Work out the finished part from the listing and answer in its coordinate system (mm). Face numbers are marked on the shaded views. Give positions to 0.01 mm unless a question says otherwise; leave off trailing zeros. Order: outer loops, then holes, each group sorted by start corner. A loop starts at its lowest first (then second) coordinate and runs counter-clockwise, first axis right, second up. Notation, with made-up numbers: (-1.75, 7) - (11.25, 7) arc R29 cw to (11.25, 32) - close; hole circle Ø7 at (71, 71). An arc over 180 degrees is marked (long way). Put each result on its own line as item: value.
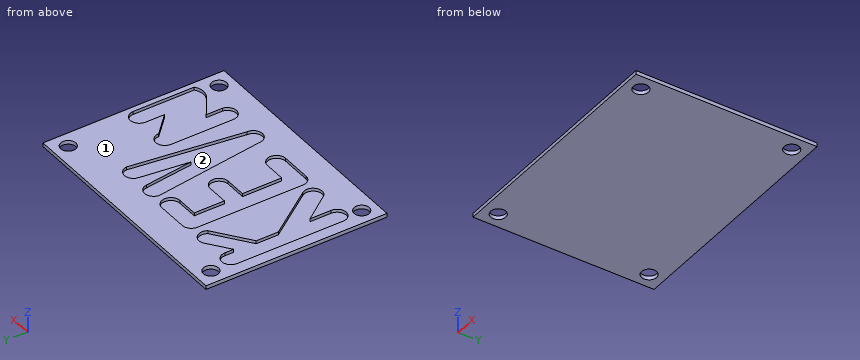
Autodesk Inventor part; units mm, degrees
ref_plane "YZ Plane" through (0, 0, 0) normal (1, 0, 0) x (0, 1, 0)
ref_plane "XZ Plane" through (0, 0, 0) normal (0, 1, 0) x (-1, 0, 0)
ref_plane "XY Plane" through (0, 0, 0) normal (0, 0, 1) x (1, 0, 0)
sketch "Sketch1" plane through (0, 0, 0) normal (0, 0, 1) x (1, 0, 0)
  line L0 (0, 0) -> (203.2, 0)
  line L1 (203.2, 0) -> (203.2, -152.4)
  line L2 (203.2, -152.4) -> (0, -152.4)
  line L3 (0, -152.4) -> (0, 0)
  line L4 (0, 0) -> (12.7, 0)
  line L5 (0, -12.7) -> (0, 0)
  line L6 (0, -152.4) -> (0, -139.7)
  line L7 (203.2, 0) -> (190.5, 0)
  line L8 (203.2, -152.4) -> (203.2, -139.7)
  circle A0 centre (12.7, -12.7) radius 6.35
  circle A1 centre (190.5, -12.7) radius 6.35
  circle A2 centre (190.5, -139.7) radius 6.35
  circle A3 centre (12.7, -139.7) radius 6.35
extrude "Extrusion1" add sketch "Sketch1" along normal blind 3.175
sketch "Sketch2" plane through (0, 0, 3.175) normal (0, 0, 1) x (1, 0, 0)
  arc A0 (24.817, -32.5655) -> (9.577, -32.5655) centre (17.197, -32.5655) ccw
  arc A1 (9.577, -122.0402) -> (24.817, -122.0402) centre (17.197, -122.0402) ccw
  line L0 (9.577, -32.5655) -> (9.577, -122.0402)
  line L1 (9.577, -42.2151) -> (9.577, -32.5655)
  arc A2 (53.0983, -37.3903) -> (42.7617, -26.7428) centre (46.6851, -33.275) ccw
  arc A3 (49.095, -40.7739) -> (42.7617, -26.7428) centre (46.7521, -33.3865) ccw
  line L2 (42.7617, -26.7428) -> (24.817, -40.0522)
  line L3 (53.0983, -37.3903) -> (24.3404, -58.7199)
  arc A4 (42.2851, -127.8629) -> (53.0983, -117.2154) centre (47.2004, -122.0402) ccw
  line L4 (53.0983, -117.2154) -> (24.3404, -77.3028)
  line L5 (42.2851, -127.8629) -> (24.817, -104.3113)
  line L6 (24.817, -104.3113) -> (24.817, -122.0402)
  line L7 (24.3404, -58.7199) -> (24.3404, -77.3028)
  line L8 (24.817, -40.0522) -> (24.817, -32.5655)
  line L9 (60.5227, -33.6636) -> (60.5227, -122.5636)
  line L10 (68.1427, -130.1836) -> (93.5427, -130.1836)
  line L11 (93.5427, -114.9436) -> (75.7627, -114.9436)
  line L12 (68.1427, -26.0436) -> (93.5427, -26.0436)
  line L13 (93.5427, -41.2836) -> (75.7627, -41.2836)
  arc A5 (68.1427, -26.0436) -> (60.5227, -33.6636) centre (68.1427, -33.6636) ccw
  arc A6 (60.5227, -122.5636) -> (68.1427, -130.1836) centre (68.1427, -122.5636) ccw
  arc A7 (93.5427, -130.1836) -> (93.5427, -114.9436) centre (93.5427, -122.5636) ccw
  arc A8 (93.5427, -41.2836) -> (93.5427, -26.0436) centre (93.5427, -33.6636) ccw
  arc A9 (93.5427, -81.8927) -> (93.5427, -66.6527) centre (93.5427, -74.2727) ccw
  line L14 (93.5427, -66.6527) -> (75.7627, -66.6527)
  line L15 (93.5427, -81.8927) -> (75.7627, -81.8927)
  line L16 (75.7627, -41.2836) -> (75.7627, -66.6527)
  line L17 (75.7627, -81.8927) -> (75.7627, -114.9436)
  line L18 (147.1171, -32.5701) -> (134.4171, -125.4887)
  line L19 (106.4768, -32.5655) -> (119.2541, -126.5682)
  line L20 (121.6953, -32.0671) -> (126.8219, -72.9902)
  line L21 (126.8219, -72.9902) -> (131.9604, -32.2167)
  arc A10 (147.1171, -32.5701) -> (131.9604, -32.2167) centre (139.5207, -33.1695) ccw
  arc A11 (119.2541, -126.5682) -> (134.4171, -125.4887) centre (126.801, -125.5424) ccw
  arc A12 (121.6953, -32.0671) -> (106.4768, -32.5655) centre (114.109, -33.0174) ccw
  line L22 (151.8189, -72.9902) -> (151.8189, -126.5682)
  arc A13 (167.0589, -72.9902) -> (151.8189, -72.9902) centre (159.4389, -72.9902) ccw
  arc A14 (151.8189, -125.6862) -> (167.0589, -126.5682) centre (159.4644, -125.6862) ccw
  line L23 (198.7066, -72.9518) -> (198.7066, -124.1784)
  line L24 (184.3126, -124.8116) -> (167.0589, -113.0447)
  line L25 (183.4405, -72.9518) -> (183.4405, -89.0244)
  line L26 (183.4405, -89.0244) -> (167.0589, -72.9902)
  line L27 (167.0589, -113.0447) -> (167.0589, -126.5682)
  arc A15 (198.7066, -72.9518) -> (183.4405, -72.9518) centre (191.0735, -72.9518) ccw
  arc A16 (184.3126, -124.8116) -> (198.7066, -124.1784) centre (191.0866, -114.8789) ccw
  point P0 (0, 0)
emboss "Emboss1" sketch "Sketch2" operation cut depth 2.54 direction (0, 0, -1)
properties part number "NamePlate"
(1) Section D-D, the plane y = -96 is taken. Write down the section's boundary in (x, z) (3 decimals), then the cut area to 3 significant figures.
Geometry check:
outline: (0, 0) - (203.2, 0) - (203.2, 3.175) - (198.707, 3.175) - (198.707, 0.635) - (151.819, 0.635) - (151.819, 3.175) - (138.448, 3.175) - (138.448, 0.635) - (115.099, 0.635) - (115.099, 3.175) - (75.763, 3.175) - (75.763, 0.635) - (60.523, 0.635) - (60.523, 3.175) - (37.812, 3.175) - (37.812, 0.635) - (9.577, 0.635) - (9.577, 3.175) - (0, 3.175) - close
area: 356 mm²
(2) Straight lines are drawn through the part: line 1 (X direction, y = -12, z = 0.75); line 2 (Y direction, x = 190.5, z = 2.25); line 3 (X direction, y = -145, z = 1.5). For each, find the intervals that lie inside material, in ascending order.
Geometry check:
line 1: x = 0 to 6.39, 19.01 to 184.19, 196.81 to 203.2
line 2: y = -152.4 to -146.05, -133.35 to -126.89, -65.34 to -19.05, -6.35 to 0
line 3: x = 0 to 9.2, 16.2 to 187, 194 to 203.2
(3) Section B-B, the plane x = 187.5 is taken. Write down the section's boundary in (y, z) (3 decimals), then the cut area to 3 significant figures.
Geometry check:
outline: (-152.4, 0) - (-145.297, 0) - (-145.297, 3.175) - (-152.4, 3.175) - close; (-134.103, 0) - (-18.297, 0) - (-18.297, 3.175) - (-66.207, 3.175) - (-66.207, 0.635) - (-126.354, 0.635) - (-126.354, 3.175) - (-134.103, 3.175) - close; (-7.103, 0) - (0, 0) - (0, 3.175) - (-7.103, 3.175) - close
area: 260 mm²
(4) Determine the mould class of the marked faces 1 and 2 for opening direction Y: pulls with the +Y half, pulls with the -Y half, needs draft (parallel to the pull), parting line crosses it, or undercut.
Geometry check:
face 1: needs draft
face 2: undercut
(5) Section A-A, the plane y = -139.7 is taken. Write down the section's boundary in (x, z) (3 decimals), then the cut area to 3 significant figures.
Geometry check:
outline: (0, 0) - (6.35, 0) - (6.35, 3.175) - (0, 3.175) - close; (19.05, 0) - (184.15, 0) - (184.15, 3.175) - (19.05, 3.175) - close; (196.85, 0) - (203.2, 0) - (203.2, 3.175) - (196.85, 3.175) - close
area: 565 mm²
(6) Given pin 1 (7.5 mm diameter, centred on x = 12.7, y = -139.7, fed in from +Z), flat-ended and moving along its own axis, determine where the tip first touches the part or whether it passes through.
Geometry check:
pin 1: passes through
(7) Section C-C, the plane x = 91 is taken. Write down the section's boundary in (y, z) (3 decimals), then the cut area to 3 significant figures.
Geometry check:
outline: (-152.4, 0) - (0, 0) - (0, 3.175) - (-26.044, 3.175) - (-26.044, 0.635) - (-41.284, 0.635) - (-41.284, 3.175) - (-66.653, 3.175) - (-66.653, 0.635) - (-81.893, 0.635) - (-81.893, 3.175) - (-114.944, 3.175) - (-114.944, 0.635) - (-130.184, 0.635) - (-130.184, 3.175) - (-152.4, 3.175) - close
area: 368 mm²
